Design review of the part built by this model. Coordinates are the model's own, in mm. Face numbers are marked on the shaded views. Round coordinates to 2 decimals unless told otherwise and drop trailing zeros. Order: outer loops, then holes, each group sorted by start corner. A loop starts at its lowest first (then second) coordinate and runs counter-clockwise, first axis right, second up.
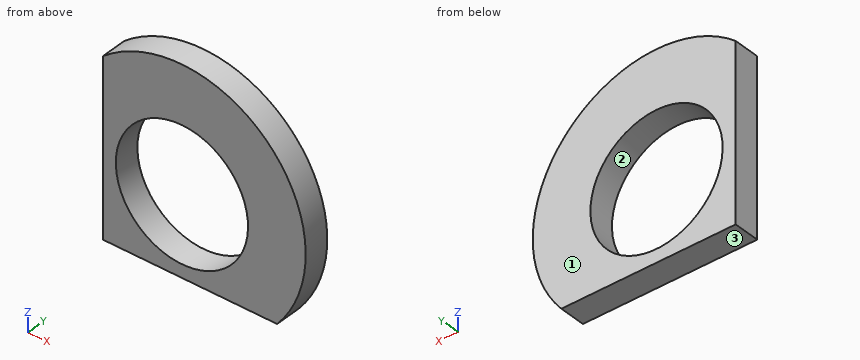
from build123d import *

# Parameters (mm, degrees)
SKETCH_1_R          = 19
SKETCH_1_R_2        = 10.15
EXTRUDE_2_DEPTH     = 4
SKETCH_3_W          = 38
SKETCH_3_H          = 10
CUT_EXTRUDE_8_DEPTH = 28.166155414
SKETCH_4_W          = 10
SKETCH_4_H          = 31.15
CUT_EXTRUDE_9_DEPTH = 28.166155414


with BuildPart() as part:
    # 草图1 → 凸台-拉伸2 (new body)
    with BuildSketch(Plane(origin=(0, 0, 0), x_dir=(1, 0, 0), z_dir=(0, 1, 0))):
        with Locations(Location((0, 0, 0), (0, 0, 270))):
            Circle(SKETCH_1_R)
        with Locations(Location((0, 0, 0), (0, 0, 270))):
            Circle(SKETCH_1_R_2, mode=Mode.SUBTRACT)
    extrude(amount=EXTRUDE_2_DEPTH)

    # 草图3 → 切除-拉伸8 (cut, through all)
    with BuildSketch(Plane(origin=(0, 4, 0), x_dir=(1, 0, 0), z_dir=(0, 1, 0))):
        with Locations((0, 17.15)):
            Rectangle(SKETCH_3_W, SKETCH_3_H)
    extrude(amount=-CUT_EXTRUDE_8_DEPTH, mode=Mode.SUBTRACT)

    # 草图4 → 切除-拉伸9 (cut, through all)
    with BuildSketch(Plane(origin=(0, 4, 0), x_dir=(1, 0, 0), z_dir=(0, 1, 0))):
        with Locations((-17.15, -3.425)):
            Rectangle(SKETCH_4_W, SKETCH_4_H)
    extrude(amount=-CUT_EXTRUDE_9_DEPTH, mode=Mode.SUBTRACT)


solid = part.part
1) Take a section at B-B on z = 0. Give the boundary of the cut face in (x, y), plus the area to 3 significant figures.
Results:
outline: (-12.15, 0) - (-10.15, 0) - (-10.15, 4) - (-12.15, 4) - close; (10.15, 0) - (19, 0) - (19, 4) - (10.15, 4) - close
area: 43.4 mm2
2) Take a section at D-D on x = 13.5. Give the boundary of the cut face in (y, z), plus the area to 3 significant figures.
Results:
outline: (0, -12.15) - (4, -12.15) - (4, 13.37) - (0, 13.37) - close
area: 102 mm2
3) The part is to be moulded in two halves that separate along Z. For the marked faces 1, 2 and 3, say which applies: released by +Z, released by -Z, zero draft, split by the parting line, or undercut.
Results:
face 1: zero draft
face 2: undercut
face 3: released by -Z
4) Clearance check with a flat-ended pin moving along its axis: P1, Ø1, axis at y = 2.5, z = 3.5, coming from the +X side. State where the tip first meets the part, or that it passes through.
Results:
P1: stops at x = 18.76
5) Take a section at A-A on x = 1. Give the boundary of the cut face in (y, z), plus the area to 3 significant figures.
Results:
outline: (0, -12.15) - (4, -12.15) - (4, -10.1) - (0, -10.1) - close; (0, 10.1) - (4, 10.1) - (4, 18.97) - (0, 18.97) - close
area: 43.7 mm2
6) To check wall thickness, follow line 1 along X through (y, z) = (2.4, 0); line 2 along X through (y, z) = (1.8, 7); line 3 along Z through (x, y) = (3.5, 3.1). State the ranges of each line that lie inside material, in increasing order.
Results:
line 1: x = -12.15 to -10.15, 10.15 to 19
line 2: x = -12.15 to -7.35, 7.35 to 17.66
line 3: z = -12.15 to -9.53, 9.53 to 18.67
7) Take a section at C-C on y = 1.1. Give the boundary of the cut face in (x, z).
Results:
outline: (-12.15, -12.15) - (14.61, -12.15) arc R19 ccw to (-12.15, 14.61) - close; hole circle Ø20.3 at (0, 0)
